The model under review builds one solid part; all positions refer to its coordinate system, in mm. A direction names the side the tool comes from. Round coordinates to 2 decimals unless told otherwise and drop trailing zeros. Order: outer loops, then holes, each group sorted by start corner. A loop starts at its lowest first (then second) coordinate and runs counter-clockwise, first axis right, second up.
1) Consider section A-A (x = 121.5). Give the boundary of the cut face in (y, z), then the cut area to 3 significant figures.
2) Consider section C-C (z = 148.5). Give the boundary of the cut face in (x, y), then the cut area to 3 significant figures.
3) Clearance check with flat-ended pins moving along their axes: P1, Ø1, axis at x = 138.5, y = 108.5, coming from the -Z side; P2, Ø5, axis at y = -44, z = 244, coming from the -X side; P3, Ø3, axis at x = -40.5, z = 247, coming from the +Y side. State where each tip first meets the part, or that it passes through.
4) Machinability: for faces 1 (the face through (-3, 3, 400)), 2 (the face through (-180, 168, 122)), 3 (the face through (-168, -180, 316)), which of the approach directions +Z, -Z, +X, -X, +Y, -Y give a long, thin tool a straight path to every point of the face, cutting with its end or side? Answer none if there is none.
5) To check wall thickness, follow L1, parallel to Y at x = 156, z = 368; L2, parallel to Z at x = 57, y = -90.5. State the ranges of each line that lie inside material, in increasing order.
6) Mouldability with a two-part tool opening along Y and no side actions: class faces 4 (the face through (-183, 182, 0)), 5 (the face through (-164, 200, 231)), 6 (the face through (168, 180, 316)), 7 (the face through (167, -180, 316)) as pulls with the +Y half, pulls with the -Y half, needs draft (parallel to the pull), parting line crosses it, or undercut.
from build123d import *

# Parameters (mm, degrees)
F1_W     = 400
F1_H     = 400
F2_DEPTH = 20
F4_DEPTH = 380
F6_W     = 360
F6_H     = 360
F7_DEPTH = 10


with BuildPart() as f2:
    # F1 (on offset) → F2 (new body)
    with BuildSketch(Plane.XY.offset(400)):
        Rectangle(F1_W, F1_H)
    extrude(amount=-F2_DEPTH)

    # F3 (on face) → F4 (join, through all)
    with BuildSketch(Plane(origin=(0, 0, 380), x_dir=(1, 0, 0), z_dir=(0, 0, -1))):
        Polygon((-155, 200), (-200, 200), (-200, 155), (-180, 155), (-180, 180), (-155, 180), align=None)
        Polygon((155, 180), (180, 180), (180, 155), (200, 155), (200, 200), (155, 200), align=None)
        Polygon((200, -200), (200, -155), (180, -155), (180, -180), (155, -180), (155, -200), align=None)
        Polygon((-180, -180), (-180, -155), (-200, -155), (-200, -200), (-155, -200), (-155, -180), align=None)
    extrude(amount=F4_DEPTH)

    # F6 (on offset) → F7 (join)
    with BuildSketch(Plane.XY.offset(250)):
        Rectangle(F6_W, F6_H)
    extrude(amount=-F7_DEPTH)


solid = f2.part
Answer below:
1. outline: (-200, 380) - (200, 380) - (200, 400) - (-200, 400) - close; (-180, 240) - (180, 240) - (180, 250) - (-180, 250) - close
1. area: 11,600 mm2
2. outline: (-200, -200) - (-155, -200) - (-155, -180) - (-180, -180) - (-180, -155) - (-200, -155) - close; (-200, 155) - (-180, 155) - (-180, 180) - (-155, 180) - (-155, 200) - (-200, 200) - close; (155, -200) - (200, -200) - (200, -155) - (180, -155) - (180, -180) - (155, -180) - close; (155, 180) - (180, 180) - (180, 155) - (200, 155) - (200, 200) - (155, 200) - close
2. area: 5,600 mm2
3. P1: stops at z = 240
3. P2: stops at x = -180
3. P3: stops at y = 180
4. face 1: +Z, +X, -X, +Y, -Y
4. face 2: -Z
4. face 3: none
5. L1: y = -200 to -180, 180 to 200
5. L2: z = 240 to 250, 380 to 400
6. face 4: needs draft
6. face 5: pulls with the +Y half
6. face 6: undercut
6. face 7: undercut
